Geometry check sheet. Reference: the model listing, model coordinates, mm. Face numbers are marked on the shaded views. A direction names the side the tool comes from. Round coordinates to 2 decimals unless told otherwise and drop trailing zeros. Order: outer loops, then holes, each group sorted by start corner. A loop starts at its lowest first (then second) coordinate and runs counter-clockwise, first axis right, second up.
(1) Draft check along Y on the marked faces 1, 2 and 3. Enter one of: pulls with the +Y half, pulls with the -Y half, needs draft (parallel to the pull), parting line crosses it, or undercut.
(2) Cross-section at A-A on z = -7. Enter the section's corners in (x, y), and give its area (3 significant figures).
(3) Gauge pin test, flat ends, axial feed: P1, Ø5, axis at x = -0.5, z = -0.5, coming from the -Y side; P2, Ø2.5, axis at y = -2.5, z = -7, coming from the -X side; P3, Ø11, axis at x = 4, y = 11.5, coming from the +Z side. Record the tip position at first contact, or that the pin passes through.
(4) Cross-section at B-B on y = 3.25. Enter the section's corners in (x, z).
(5) Set-up check for the marked faces 4, 5 and 6: record each of +Z, -Z, +X, -X, +Y, -Y from which the full face is reachable in a straight line by a thin tool's end or side.
(6) Thickness scan on L1, parallel to Y at x = 5, z = 7.75; L2, parallel to Y at x = 2.5, z = -5; L3, parallel to X at y = 13.75, z = -14.25. Record the ranges inside material, lowest first.
(7) Cross-section at C-C on z = 1. Enter the section's corners in (x, y).
(8) Cross-section at D-D on x = 5.75. Enter the section's corners in (y, z).
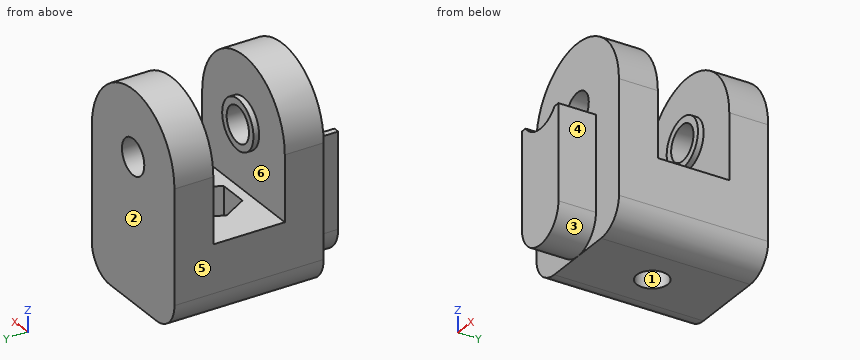
from build123d import *

# Parameters (mm, degrees)
SKETCH1_R           = 2.5
BOSS_EXTRUDE1_DEPTH = 21.1
SKETCH2_W           = 18.5
SKETCH2_H           = 10.1
CUT_EXTRUDE1_DEPTH  = 35.459541494
BOSS_EXTRUDE3_DEPTH = 5.3
SKETCH4_R           = 3.5
SKETCH4_R_2         = 2.5
BOSS_EXTRUDE4_DEPTH = 0.8
FILLET1_R           = 4
CUT_EXTRUDE2_DEPTH  = 7
SKETCH6_R           = 2.2
CUT_EXTRUDE3_DEPTH  = 7


with BuildPart() as part:
    # Sketch1 → Boss-Extrude1 (new body)
    with BuildSketch(Plane(origin=(0, 0, 0), x_dir=(1, 0, 0), z_dir=(0, 1, 0))):
        with BuildLine():
            Line((-9.25, 0), (-9.25, 20))
            Line((-9.25, 20), (9.25, 20))
            Line((9.25, 20), (9.25, 0))
            ThreePointArc((9.25, 0), (0, -9.25), (-9.25, 0))
        make_face()
        with Locations(Location((0, 0, 0), (0, 0, 270))):
            Circle(SKETCH1_R, mode=Mode.SUBTRACT)
    extrude(amount=BOSS_EXTRUDE1_DEPTH)

    # Sketch2 → Cut-Extrude1 (cut, through all)
    with BuildSketch(Plane(origin=(9.25, 0, 0), x_dir=(0, 0, -1), z_dir=(1, 0, 0))):
        with Locations((0, 10.55)):
            Rectangle(SKETCH2_W, SKETCH2_H)
    extrude(amount=-CUT_EXTRUDE1_DEPTH, mode=Mode.SUBTRACT)

    # Sketch3 → Boss-Extrude3 (add)
    with BuildSketch(Plane.XZ):
        with BuildLine():
            Line((4.1, -2.5), (4.1, -15.9))
            ThreePointArc((4.1, -15.9), (0, -20), (-4.1, -15.9))
            Line((-4.1, -15.9), (-4.1, -2.5))
            Line((-4.1, -2.5), (-3.249615362, -2.5))
            ThreePointArc((-3.249615362, -2.5), (0, -4.1), (3.249615362, -2.5))
            Line((3.249615362, -2.5), (4.1, -2.5))
        make_face()
    extrude(amount=BOSS_EXTRUDE3_DEPTH)

    # Sketch4 → Boss-Extrude4 (add)
    with BuildSketch(Plane(origin=(0, 5.5, 0), x_dir=(1, 0, 0), z_dir=(0, 1, 0))):
        with Locations(Location((0, 0, 0), (0, 0, 90))):
            Circle(SKETCH4_R)
        with Locations(Location((0, 0, 0), (0, 0, 270))):
            Circle(SKETCH4_R_2, mode=Mode.SUBTRACT)
    boss_extrude4 = extrude(amount=BOSS_EXTRUDE4_DEPTH)

    # Mirror1: Boss-Extrude4 across plane
    add(boss_extrude4.mirror(Plane.ZX.offset(10.55)))

    # Fillet1
    fillet1_edges = [part.edges().sort_by_distance(p)[0] for p in [
        (-9.25, 10.55, -20),
        (9.25, 10.55, -20),
    ]]
    fillet(fillet1_edges, radius=FILLET1_R)

    # Sketch5 → Cut-Extrude2 (cut)
    with BuildSketch(Plane.XY.offset(-9.25)):
        Polygon((2.078460969, 6.95), (4.156921938, 10.55), (2.078460969, 14.15), (-2.078460969, 14.15), (-4.156921938, 10.55), (-2.078460969, 6.95), align=None)
    extrude(amount=-CUT_EXTRUDE2_DEPTH, mode=Mode.SUBTRACT)

    # Sketch6 → Cut-Extrude3 (cut)
    with BuildSketch(Plane.XY.offset(-16.25)):
        with Locations((0, 10.55)):
            Circle(SKETCH6_R)
    extrude(amount=-CUT_EXTRUDE3_DEPTH, mode=Mode.SUBTRACT)


solid = part.part
Found:
1. face 1: undercut
1. face 2: pulls with the +Y half
1. face 3: needs draft
2. outline: (-9.25, 0) - (-4.1, 0) - (-4.1, -5.3) - (4.1, -5.3) - (4.1, 0) - (9.25, 0) - (9.25, 5.5) - (-9.25, 5.5) - close; (-9.25, 15.6) - (9.25, 15.6) - (9.25, 21.1) - (-9.25, 21.1) - close
2. area: 247 mm2
3. P1: stops at y = 0
3. P2: stops at x = -4.1
3. P3: stops at z = 9.24
4. outline: (-9.25, -16) arc R4 ccw to (-5.25, -20) - (5.25, -20) arc R4 ccw to (9.25, -16) - (9.25, 0) arc R9.25 ccw to (-9.25, 0) - close; hole circle Ø5 at (0, 0)
5. face 4: +Z, -Z, +X, -Y
5. face 5: +Z, -Z, -X, +Y, -Y
5. face 6: none
6. L1: y = 0 to 5.5, 15.6 to 21.1
6. L2: y = -5.3 to 5.5, 15.6 to 21.1
6. L3: x = -9.25 to -2.31, 2.31 to 9.25
7. outline: (-9.2, 0) - (-2.29, 0) - (-2.29, 6.3) - (-3.35, 6.3) - (-3.35, 5.5) - (-9.2, 5.5) - close; (-9.2, 15.6) - (-3.35, 15.6) - (-3.35, 14.8) - (-2.29, 14.8) - (-2.29, 21.1) - (-9.2, 21.1) - close; (2.29, 0) - (9.2, 0) - (9.2, 5.5) - (3.35, 5.5) - (3.35, 6.3) - (2.29, 6.3) - close; (2.29, 14.8) - (3.35, 14.8) - (3.35, 15.6) - (9.2, 15.6) - (9.2, 21.1) - (2.29, 21.1) - close
8. outline: (0, -19.97) - (21.1, -19.97) - (21.1, 7.25) - (15.6, 7.25) - (15.6, -9.25) - (5.5, -9.25) - (5.5, 7.25) - (0, 7.25) - close
